For this review, take the finished solid that the model builds, in its own axes (mm). Give positions to 0.01 mm unless a question says otherwise; leave off trailing zeros. Write each loop counter-clockwise with the first axis right and the second up, starting at its lowest first coordinate (ties: lowest second). Pieces come first, ordered by that corner, then holes.
Q1. We need section A-A (y = 0.3). Write out the cut boundary in (x, z), then the cut area to 3 significant figures.
Q2. Mouldability with a two-part tool opening along X and no side actions: class faces 1 (the cylindrical face through (-0.86, -0.016, 3.874)), 2 (the flat face through (-4, -1.389, -2)), 3 (the cylindrical face through (4.96, -0.94, -1.56)) as released by +X, released by -X, zero draft, split by the parting line, or undercut.
Q3. Insertion check: P1, Ø5, axis at x = 2, z = 3, coming from the +Y side; P2, Ø1.5, axis at y = -1, z = 2, coming from the +X side. Each pin has a flat end and moves straight along its axis. Give the tip position at first contact, or say it passes through.
Q4. For line 1 (X direction, y = -1.2, z = 2.75); line 2 (Z direction, x = 0, y = -0.05); line 3 (Z direction, x = 0, y = -0.3), list the stretches that pass through material, from the lowest coordinate up.
```python
from build123d import *

# Parameters (mm, degrees)
CHAMFER1_SIZE = 0.25
FILLET1_R     = 0.2


with BuildPart() as part:
    # Sketch1 → Revolve1 (revolve)
    with BuildSketch(Plane.XY):
        with BuildLine():
            Line((3.96875, 1.3890625), (3.96875, -1.3890625))
            Line((3.96875, -1.3890625), (5.2, -1.3890625))
            Line((5.2, -1.3890625), (5.2, -0.594165218))
            Line((5.2, -0.594165218), (4.841347672, -0.474161828))
            ThreePointArc((4.841347672, -0.474161828), (4.5, 0), (4.841347672, 0.474161828))
            Line((4.841347672, 0.474161828), (5.2, 0.594165218))
            Line((5.2, 0.594165218), (5.2, 1.3890625))
            Line((5.2, 1.3890625), (3.96875, 1.3890625))
        make_face()
    revolve(axis=Axis((0, 0, 0), (0, 1, 0)))

    # Chamfer1
    chamfer1_edges = [part.edges().sort_by_distance(p)[0] for p in [
        (-3.96875, 1.3890625, 0),
        (-5.2, 1.3890625, 0),
        (-5.2, -1.3890625, 0),
        (-3.96875, -1.3890625, 0),
    ]]
    chamfer(chamfer1_edges, length=CHAMFER1_SIZE)

    # Fillet1
    fillet1_edges = [part.edges().sort_by_distance(p)[0] for p in [
        (-5.2, 0.594165218, 0),
        (-5.2, -0.594165218, 0),
    ]]
    fillet(fillet1_edges, radius=FILLET1_R)


solid = part.part
```
Computed:
1. outline: circle Ø9.2 at (0, 0); hole circle Ø7.94 at (0, 0)
1. area: 17.0 mm2
2. face 1: undercut
2. face 2: zero draft
2. face 3: split by the parting line
3. P1: stops at y = 1.39
3. P2: stops at x = 5.05
4. line 1: x = -4.34 to -2.95, 2.95 to 4.34
4. line 2: z = -4.5 to -3.97, 3.97 to 4.5
4. line 3: z = -4.6 to -3.97, 3.97 to 4.6
